Read the model definition and answer for the solid it produces. Units are mm, in the model's axes. A direction names the side the tool comes from. Round coordinates to 2 decimals unless told otherwise and drop trailing zeros. Write each loop counter-clockwise with the first axis right and the second up, starting at its lowest first coordinate (ties: lowest second). Pieces come first, ordered by that corner, then holes. Notation, with made-up numbers: (-4.75, 66) -> (29.25, 66) arc R18 cw to (29.25, 77) -> close; hole circle Ø9 at (86.25, 10.25). An arc over 180 degrees is marked (long way). Return JSON: item names as keys, results as strings. Group by question number.
(1) Given pin 1 (4 mm diameter, centred on y = 4.5, z = 7.5, fed in from +X); pin 2 (3.5 mm diameter, centred on x = -0.5, z = 12.5, fed in from -Y); pin 3 (2 mm diameter, centred on x = -1, z = 11.5, fed in from +Y), each flat-ended and moving along its own axis, determine where each tip first touches the part or whether it passes through.
(2) Straight lines are drawn through the part: line 1 (Z direction, x = 6, y = 14); line 2 (Y direction, x = 0.75, z = 8.25); line 3 (Y direction, x = 3.25, z = 4). For each, find the intervals that lie inside material, in ascending order.
(3) A cutting plane is placed at D-D on y = 13. Give the vertices of the cut face in (x, z) (3 decimals), then the cut area to 3 significant figures.
(4) A cutting plane is placed at A-A on y = -4. Give the vertices of the cut face in (x, z) (3 decimals).
(5) A cutting plane is placed at B-B on z = 9.25. Give the vertices of the cut face in (x, y), then the cut area to 3 significant figures.
(6) A cutting plane is placed at C-C on x = -1.5. Give the vertices of the cut face in (y, z).
(7) For faces 1 (the flat face through (0, -12.5, 10)), 2 (the flat face through (0, 12.5, 10)), 3 (the flat face through (-3.5, 0, 10)), determine the directions among +Z, -Z, +X, -X, +Y, -Y from which every point of the face is accessible in a straight line to the end or side of a thin tool.
```python
from build123d import *

# Parameters (mm, degrees)
RESSALTO_EXTRUS_O1_DEPTH = 5.4
CHANFRO1_SIZE            = 6
ESBO_O2_W                = 7
ESBO_O2_H                = 25
RESSALTO_EXTRUS_O2_DEPTH = 10
CHANFRO2_SIZE            = 6
CHANFRO2_SIZE_2          = 2.183821406


with BuildPart() as part:
    # Esboço1 → Ressalto-extrusão1 (new body)
    with BuildSketch(Plane.XY):
        Polygon((-14.825, -17.5), (0, -24.5), (14.825, -17.5), (14.825, 17.5), (-14.825, 17.5), align=None)
    extrude(amount=RESSALTO_EXTRUS_O1_DEPTH)

    # Chanfro1
    # the kernel refuses this chamfer: 6 mm, written as the material it takes off along each edge
    with BuildSketch(Plane(origin=(-13.952897525, -31.088214683, 5.4), x_dir=(0.01173996035917391, -0.024863558903536174, -0.9996219169112968), z_dir=(0.9042650014643773, 0.4269716701686773, 0)), Plane(origin=(-28.777897525, -10.911785317, 5.4), x_dir=(-0.01173996035917391, -0.024863558903536174, -0.9996219169112968), z_dir=(0.9042650014643773, -0.4269716701686773, 0))) as chanfro1_piece_1:
        Polygon((CHANFRO1_SIZE * 0.999621916911, CHANFRO1_SIZE * 0.0274958766106), (-CHANFRO1_SIZE * 0.0274958766106, CHANFRO1_SIZE * 0.999621916911), (0, 0), align=None)
    extrude(amount=47.254726193, mode=Mode.SUBTRACT)

    # Esboço2 → Ressalto-extrusão2 (add)
    with BuildSketch(Plane.XY.offset(5.4)):
        Rectangle(ESBO_O2_W, ESBO_O2_H)
    extrude(amount=RESSALTO_EXTRUS_O2_DEPTH)

    # Chanfro2
    # the kernel refuses this chamfer: 6, 2.183821406 mm, written as the material it takes off along each edge
    with BuildSketch(Plane(origin=(30.390168395, 17.5, 5.4), x_dir=(0, 0.013184058198645722, -0.9999130865277315), z_dir=(-1, 0, 0))) as chanfro2_piece_1:
        Polygon((CHANFRO2_SIZE * 0.999913086528, CHANFRO2_SIZE * 0.0131840581986), (-CHANFRO2_SIZE_2 * 0.0131840581962, CHANFRO2_SIZE_2 * 0.999913086343), (0, 0), align=None)
    extrude(amount=60.780336791, mode=Mode.SUBTRACT)


solid = part.part
```
Checks:
{
 "1": {"pin 1": "stops at x = 3.5", "pin 2": "stops at y = -12.5", "pin 3": "stops at y = 12.5"},
 "2": {"line 1": "z = 0 to 5.4", "line 2": "y = -12.5 to 12.5", "line 3": "y = -17.88 to 15.83"},
 "3": {"outline": "(-14.825, 0) -> (14.825, 0) -> (14.825, 5.4) -> (-14.825, 5.4) -> close", "area": "160 mm^2"},
 "4": {"outline": "(-14.825, 0) -> (14.825, 0) -> (14.825, 5.4) -> (3.5, 5.4) -> (3.5, 15.4) -> (-3.5, 15.4) -> (-3.5, 5.4) -> (-14.825, 5.4) -> close"},
 "5": {"outline": "(-3.5, -12.5) -> (3.5, -12.5) -> (3.5, 12.5) -> (-3.5, 12.5) -> close", "area": "175 mm^2"},
 "6": {"outline": "(-23.13, 0) -> (17.28, 0) -> (15.32, 5.4) -> (12.5, 5.4) -> (12.5, 15.4) -> (-12.5, 15.4) -> (-12.5, 5.4) -> (-17.16, 5.4) -> close"},
 "7": {"face 1": "+Z, +X, -X, -Y", "face 2": "+Z, +X, -X, +Y", "face 3": "+Z, -X, +Y, -Y"}
}
